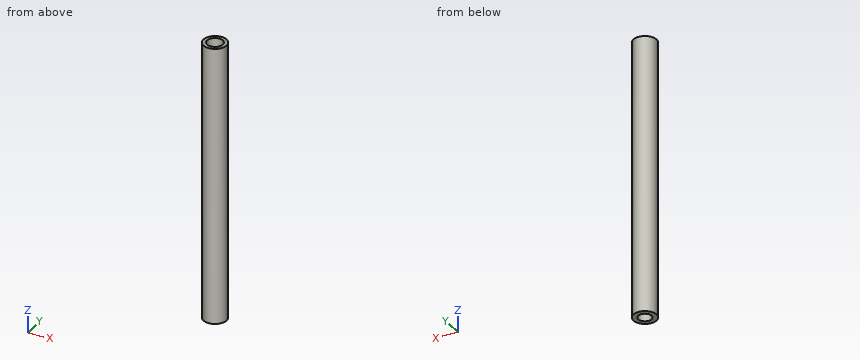
```python
from build123d import *

# Parameters (mm, degrees)
F0_R     = 38.1
F0_R_2   = 22.225
F1_DEPTH = 914.4
F3_R     = 26
F3_R_2   = 22.225
F4_DEPTH = 152.4
F5_R     = 24.09825
F6_DEPTH = 6.35


# Not quite as in the source:
# - a feature names something its author has since deleted; it is built from what else it names


with BuildPart() as f1:
    # F0 (on Top) → F1 (new body)
    with BuildSketch(Plane.XY):
        Circle(F0_R)
        Circle(F0_R_2, mode=Mode.SUBTRACT)
    extrude(amount=F1_DEPTH)

    # F3 (on face) → F4 (cut)
    with BuildSketch(Plane.XY.offset(914.4)):
        Circle(F3_R)
        Circle(F3_R_2, mode=Mode.SUBTRACT)
    extrude(amount=-F4_DEPTH, mode=Mode.SUBTRACT)

    # F5 (on face) → F6 (cut)
    with BuildSketch(Plane.XY.offset(762)):
        Circle(F5_R)
    extrude(amount=-F6_DEPTH, mode=Mode.SUBTRACT)


solid = f1.part
```
Input: part model. Units: mm. Frame: model coordinates. Coordinates: 2 decimals unless noted, no trailing zeros. Write each loop counter-clockwise with the first axis right and the second up, starting at its lowest first coordinate (ties: lowest second). Pieces come first, ordered by that corner, then holes. Notation, with made-up numbers: (-15, 19.5) -> (-3, 19.5) arc R6 ccw to (-3, 27.5) -> close; hole circle Ø6 at (-10, 34). An arc over 180 degrees is marked (long way). Answer as a JSON object with one key per item and string values.
1. First-contact query: P1, Ø14.5, axis at x = 11.5, y = 11, coming from the +Z side; P2, Ø1.5, axis at x = 8, z = 150, coming from the +Y side; P3, Ø1.5, axis at x = -21, z = 295.5, coming from the +Y side. Flat tips, straight axial feed; report the tip coordinate or a pass-through.
Result set:
{"P1": "stops at z = 755.65", "P2": "stops at y = 37.4", "P3": "stops at y = 32.27"}
2. Section A-A on x = 0. Return the cut outline in (y, z) (3 decimals), then the cut area to 3 significant figures.
Result set:
{"outline": "(-38.1, 0) -> (-22.225, 0) -> (-22.225, 755.65) -> (-24.098, 755.65) -> (-24.098, 762) -> (-26, 762) -> (-26, 914.4) -> (-38.1, 914.4) -> close; (22.225, 0) -> (38.1, 0) -> (38.1, 914.4) -> (26, 914.4) -> (26, 762) -> (24.098, 762) -> (24.098, 755.65) -> (22.225, 755.65) -> close", "area": "27,900 mm2"}
3. Section C-C on z = 244.5. Return the cut outline in (x, y) (3 decimals).
Result set:
{"outline": "circle Ø76.2 at (0, 0); hole circle Ø44.45 at (0, 0)"}
4. Material intervals for line 1 (Y direction, x = 0, z = 528) (3 decimals); line 2 (Y direction, x = 0, z = 861); line 3 (X direction, y = 7, z = 482.5), sorted ascending. Write a range as from..to.
Result set:
{"line 1": "y = -38.1..-22.225, 22.225..38.1", "line 2": "y = -38.1..-26, 26..38.1", "line 3": "x = -37.45..-21.09, 21.09..37.45"}
